from build123d import *

# Parameters (mm, degrees)
DOWELSUPPORT_DEPTH          = 1.905
DOWELSUPPORT_DEPTH_BACK     = 1.27
SKETCH3_R                   = 3.81
SKETCH5_W                   = 6.35
SKETCH5_H                   = 28.575
SLIDERDOWELSUPPORT_DEPTH    = 1.27
SLIDERDOWELCUTOUT_DEPTH     = 13.335
CUT_EXTRUDE2_DEPTH          = 29.782824115
CUT_EXTRUDE2_DEPTH_BACK     = 29.782824115
SKETCH20_W                  = 1.27
SKETCH20_H                  = 12.7
LPATTERN1_COUNT             = 2
LPATTERN1_PITCH             = 19.05
LATERALSUPPORT_DEPTH        = 1.27
SKETCH8_W                   = 6.35
SKETCH8_H                   = 3
TABSUPPORT_DEPTH            = 1.27
STRINGDOWELSUPPORT_START    = -1.27
STRINGDOWELSUPPORT_DEPTH    = 5.715
INTERSUPPORT_DEPTH          = 1.27
SKETCH10_W                  = 6.35
SKETCH10_H                  = 3
TABBASE_DEPTH               = 1.27
SKETCH12_W                  = 6.35
SKETCH12_H                  = 3
TABDRAFT_DEPTH              = 1.73
TABDRAFT_DRAFT              = 5
TABDRAFT_PROFILE_2_DEPTH    = 1.73
TABDRAFT_PROFILE_2_DRAFT    = 5
STRINGDOWELHOLES_DEPTH      = 39.922670163
STRINGDOWELHOLES_DEPTH_BACK = 1.524
SKETCH14_R                  = 1.600000102
PULLEYDOWELHOLE_DEPTH       = 2.921
FILLET1_R                   = 6.35


with BuildPart() as part:
    # Sketch3 → DowelSupport (new, two sides: drawn at the far end of the back side and taken through both)
    with BuildSketch(Plane(origin=(0, 0, 0), x_dir=(0, 0, -1), z_dir=(1, 0, 0)).offset(-DOWELSUPPORT_DEPTH_BACK)):
        with Locations((0, 24.60625)):
            Circle(SKETCH3_R)
    extrude(amount=DOWELSUPPORT_DEPTH + DOWELSUPPORT_DEPTH_BACK)

    # Sketch8 → TabSupport (add, symmetric)
    with BuildSketch(Plane(origin=(0, 0, 0), x_dir=(0, 0, -1), z_dir=(1, 0, 0))):
        with Locations((0, 21.59)):
            Rectangle(SKETCH8_W, SKETCH8_H)
        with Locations((-12.7, 21.59)):
            Rectangle(SKETCH8_W, SKETCH8_H)
    extrude(amount=TABSUPPORT_DEPTH, both=True)


with BuildPart() as body_2:
    # Sketch5 → SliderDowelSupport (new, symmetric)
    with BuildSketch(Plane(origin=(0, 0, 0), x_dir=(0, 0, -1), z_dir=(1, 0, 0))):
        Rectangle(SKETCH5_W, SKETCH5_H)
    extrude(amount=SLIDERDOWELSUPPORT_DEPTH, both=True)

    # Sketch19 → SliderDowelCutout (cut, symmetric)
    with BuildSketch(Plane(origin=(0, 0, 0), x_dir=(1, 0, 0), z_dir=(0, 1, 0))):
        with BuildLine():
            Line((1.27, 1.350000094), (1.243577144, 1.350000094))
            ThreePointArc((1.243577144, 1.350000094), (-1.068, 0), (1.243577144, -1.350000094))
            Line((1.243577144, -1.350000094), (1.27, -1.350000094))
            Line((1.27, -1.350000094), (1.27, 1.350000094))
        make_face()
    extrude(amount=SLIDERDOWELCUTOUT_DEPTH, both=True, mode=Mode.SUBTRACT)

    # Sketch20 → Cut-Extrude2 (cut, two sides: drawn at the far end of the back side and taken through both)
    with BuildSketch(Plane(origin=(1.27, 0, 0), x_dir=(0, 0, -1), z_dir=(1, 0, 0)).offset(-CUT_EXTRUDE2_DEPTH_BACK)):
        Rectangle(SKETCH20_W, SKETCH20_H)
    extrude(amount=CUT_EXTRUDE2_DEPTH + CUT_EXTRUDE2_DEPTH_BACK, mode=Mode.SUBTRACT)


with BuildPart() as lpattern1_1:
    # LPattern1: pattern copy
    add(body_2.part.moved(Location(Vector(0, 0, 1) * (1 * LPATTERN1_PITCH))))


with BuildPart() as body_4:
    # Sketch6 → LateralSupport (new, symmetric)
    with BuildSketch(Plane(origin=(0, 0, 0), x_dir=(0, 0, -1), z_dir=(1, 0, 0))):
        Polygon((7.392863577, 27.041434671), (5.805363577, 29.791065329), (8.169612929, 31.156065329), (9.523465192, 31.351124423), (10.602965192, 29.481375577), (9.757112929, 28.406434671), align=None)
    extrude(amount=LATERALSUPPORT_DEPTH, both=True)


with BuildPart() as tabsupport_piece_1:
    # of the separate pieces the step leaves, piece 1, a body of its own (tabsupport_pieces)
    add(part.part.solids().sort_by_distance((0, 24.60625, -3.81))[0])


with BuildPart() as tabsupport_piece_2:
    # of the separate pieces the step leaves, piece 2, a body of its own (tabsupport_pieces)
    add(part.part.solids().sort_by_distance((-1.27, 20.09, 9.525))[0])

    # Sketch15 → StringDowelSupport (add)
    with BuildSketch(Plane(origin=(0, 0, 0), x_dir=(0, 0, -1), z_dir=(1, 0, 0)).offset(STRINGDOWELSUPPORT_START)):
        with BuildLine():
            Line((-14.4145, 23.876), (-10.9855, 23.876))
            ThreePointArc((-10.9855, 23.876), (-8.6995, 21.59), (-10.9855, 19.304))
            Line((-10.9855, 19.304), (-14.4145, 19.304))
            ThreePointArc((-14.4145, 19.304), (-16.7005, 21.59), (-14.4145, 23.876))
        make_face()
    extrude(amount=STRINGDOWELSUPPORT_DEPTH)


with BuildPart() as body_2_1:
    add(body_2.part)

    add(lpattern1_1.part)  # InterSupport merges LPattern1_1

    add(body_4.part)  # InterSupport merges body 4

    add(tabsupport_piece_1.part)  # InterSupport merges TabSupport piece 1

    add(tabsupport_piece_2.part)  # InterSupport merges TabSupport piece 2
    # Sketch7 → InterSupport (add, symmetric)
    with BuildSketch(Plane(origin=(0, 0, 0), x_dir=(0, 0, -1), z_dir=(1, 0, 0))):
        Polygon((8.027863577, 25.941582409), (5.170363577, 30.890917591), (-1.187110053, 27.22042848), (-0.923046602, 27.310559749), (0, 24.60625), (1.42875, 22.131582409), align=None)
        Polygon((-1.42875, 27.080917591), (-1.187110053, 27.22042848), (-10.9855, 23.876), (-14.4145, 23.876), (-15.582507886, 22.531146949), (-22.225, 14.2875), (-15.875, 14.2875), (-15.875, 0), (-3.175, 0), (-3.175, 14.2875), (3.175, 14.2875), (3.175, 20.09), (0.923046602, 21.901940251), (0, 24.60625), align=None)
    extrude(amount=INTERSUPPORT_DEPTH, both=True)

    # Sketch10 → TabBase (add)
    with BuildSketch(Plane.ZY.offset(1.27)):
        with Locations((0, 21.59)):
            Rectangle(SKETCH10_W, SKETCH10_H)
        with Locations((12.7, 21.59)):
            Rectangle(SKETCH10_W, SKETCH10_H)
    extrude(amount=TABBASE_DEPTH)


with BuildPart() as tabdraft_tool:
    # Sketch12 → TabDraft (with draft: the straight prism first)
    with BuildSketch(Plane.ZY.offset(2.54)):
        with Locations((0, 21.59)):
            Rectangle(SKETCH12_W, SKETCH12_H)
    extrude(amount=TABDRAFT_DEPTH)
    # TabDraft: the draft: its side faces are tilted about the plane it starts from
    tabdraft_sides = [tabdraft_tool.faces().sort_by_distance(p)[0] for p in [
        (-3.405, 21.59, 3.175),
        (-3.405, 23.09, 0),
        (-3.405, 21.59, -3.175),
        (-3.405, 20.09, 0),
    ]]
    draft(tabdraft_sides, Plane.ZY.offset(2.54), TABDRAFT_DRAFT)


with BuildPart() as body_2_2:
    add(body_2_1.part)

    # TabDraft: add tabdraft_tool
    add(tabdraft_tool.part)


with BuildPart() as tabdraft_profile_2_tool:
    # Sketch12 → TabDraft profile 2 (with draft: the straight prism first)
    with BuildSketch(Plane.ZY.offset(2.54)):
        with Locations((12.7, 21.59)):
            Rectangle(SKETCH12_W, SKETCH12_H)
    extrude(amount=TABDRAFT_PROFILE_2_DEPTH)
    # TabDraft profile 2: the draft: its side faces are tilted about the plane it starts from
    tabdraft_profile_2_sides = [tabdraft_profile_2_tool.faces().sort_by_distance(p)[0] for p in [
        (-3.405, 21.59, 9.525),
        (-3.405, 20.09, 12.7),
        (-3.405, 21.59, 15.875),
        (-3.405, 23.09, 12.7),
    ]]
    draft(tabdraft_profile_2_sides, Plane.ZY.offset(2.54), TABDRAFT_PROFILE_2_DRAFT)


with BuildPart() as body_2_3:
    add(body_2_2.part)

    # TabDraft profile 2: add tabdraft_profile_2_tool
    add(tabdraft_profile_2_tool.part)

    # Sketch16 → StringDowelHoles (cut, two sides: drawn at the far end of the back side and taken through both)
    with BuildSketch(Plane(origin=(1.905, 0, 0), x_dir=(0, 0, -1), z_dir=(1, 0, 0)).offset(-STRINGDOWELHOLES_DEPTH_BACK)):
        with BuildLine():
            Line((-13.00760401, 20.828), (-12.39239599, 20.828))
            ThreePointArc((-12.39239599, 20.828), (-9.385499898, 21.59), (-12.39239599, 22.352))
            Line((-12.39239599, 22.352), (-13.00760401, 22.352))
            ThreePointArc((-13.00760401, 22.352), (-16.014500102, 21.59), (-13.00760401, 20.828))
        make_face()
    extrude(amount=STRINGDOWELHOLES_DEPTH + STRINGDOWELHOLES_DEPTH_BACK, mode=Mode.SUBTRACT)

    # Sketch14 → PulleyDowelHole (cut)
    with BuildSketch(Plane(origin=(1.905, 0, 0), x_dir=(0, 0, -1), z_dir=(1, 0, 0))):
        with Locations((0, 24.60625)):
            Circle(SKETCH14_R)
    extrude(amount=-PULLEYDOWELHOLE_DEPTH, mode=Mode.SUBTRACT)

    # Mirror1: body 2 across plane


with BuildPart() as body_2_4:
    add(body_2_3.part)
    add(body_2_3.part.mirror(Plane.ZX))

    # Fillet1
    fillet1_edges = [body_2_4.edges().sort_by_distance(p)[0] for p in [
        (0, -14.2875, 22.225),
        (0, 14.2875, 22.225),
    ]]
    fillet(fillet1_edges, radius=FILLET1_R)


solid = body_2_4.part
Can you work these out from the model? Positions are in its coordinate system, mm. A direction names the side the tool comes from. Coordinates: 2 decimals unless noted, no trailing zeros. Loops run counter-clockwise (first coordinate to the right, second up) from the corner with the lowest first, then second, coordinate; pieces in that order, holes last. Notation, with made-up numbers: (89.5, -17.75) - (120.5, -17.75) arc R14 cw to (120.5, 5.25) - close; hole circle Ø11 at (15, -14.75). An arc over 180 degrees is marked (long way). Put each result on its own line as item: value. Start each with the question number.
Item 1: Suppose I cut it at C-C (y = -7). Please give me the cut outline in (x, z) (3 decimals), and give its area (3 significant figures).
Item 2: Suppose I cut it at D-D (z = 15). Please give me the cut outline in (x, y) (3 decimals), and give its area (3 significant figures).
Item 3: For pin 1 (1 mm diameter, centred on x = -2, y = 22, fed in from +Z) (3 decimals); pin 2 (1.4 mm diameter, centred on x = -2, z = 1.5, fed in from -Y); pin 3 (6 mm diameter, centred on y = 25, z = 1, fed in from +X) (3 decimals), each with a flat end and sliding along its axis, tell me the tip position at first contact or that it passes through.
Item 4: Suppose I cut it at B-B (z = 19.05). Please give me the cut outline in (x, y) (3 decimals).
Item 5: Which directions (+Z, -Z, +X, -X, +Y, -Y) give clear straight access to the entire face, cutting with the end or side of a thin tool? Please do faces 1 (the face through (2, -23.876, 13)), 2 (the face through (0.018, -30.333, -5.492)), 3 (the face through (-2, 20.09, 0)), 4 (the face through (1.905, -25, -2)).
Item 6: If I drill on line 1 along Y through (x, z) = (-2.5, 0.5); line 2 along Z through (x, y) = (2, -22.5); line 3 along Z through (x, y) = (1.4, -21.59), over which ranges is the centre line in solid material (lowest first)?
Item 7: If we mould it in two halves opening along Y, with no side actions, what happens to faces 5 (the face through (0.018, 25.205, 7.093)), 6 (the face through (2.8, 21.6, 8.7)), 7 (the face through (0, -13.335, 0)), 8 (the face through (4.445, -20.6, 12.6))? For each: +Y half, -Y half, draft (parallel to the pull), parting line (faces both ways), or undercut.
Item 8: Suppose I cut it at A-A (x = 2.5). Please give me the cut outline in (y, z).
Here are the results:
1. outline: (-1.27, -3.175) - (1.27, -3.175) - (1.27, -1.35) - (1.244, -1.35) arc R1.55 cw (long way) to (1.244, 1.35) - (1.27, 1.35) - (1.27, 17.7) - (1.244, 17.7) arc R1.55 cw (long way) to (1.244, 20.4) - (1.27, 20.4) - (1.27, 22.225) - (-1.27, 22.225) - close
1. area: 52.3 mm²
2. outline: (-4.27, -22.939) - (-2.54, -23.09) - (-1.27, -23.09) - (-1.27, -23.8) - (4.445, -23.8) - (4.445, -23.079) - (0.381, -23.079) - (0.381, -20.101) - (4.445, -20.101) - (4.445, -19.38) - (1.27, -19.38) - (1.27, 19.38) - (4.445, 19.38) - (4.445, 20.101) - (0.381, 20.101) - (0.381, 23.079) - (4.445, 23.079) - (4.445, 23.8) - (-1.27, 23.8) - (-1.27, 23.09) - (-2.54, 23.09) - (-4.27, 22.939) - (-4.27, 20.241) - (-2.54, 20.09) - (-1.27, 20.09) - (-1.27, -20.09) - (-2.54, -20.09) - (-4.27, -20.241) - close
2. area: 142 mm²
3. pin 1: z = 15.875
3. pin 2: y = -23.09
3. pin 3: x = 1.905
4. outline: (-1.27, -18.228) - (1.27, -18.228) - (1.27, -13.335) - (-1.068, -13.335) - (-1.068, -6.35) - (-1.27, -6.35) - close; (-1.27, 6.35) - (-1.068, 6.35) - (-1.068, 13.335) - (1.27, 13.335) - (1.27, 18.228) - (-1.27, 18.228) - close
5. face 1: +Z, +X, -X, -Y
5. face 2: +X, -X, -Y
5. face 3: +Z, -Z, -X
5. face 4: -Z, +X, +Y, -Y
6. line 1: -23.09 to -20.09, 20.09 to 23.09
6. line 2: 8.89 to 9.67, 12.3 to 13.1, 15.73 to 16.51
6. line 3: -2.33 to 2.33, 8.7 to 9.39, 16.01 to 16.7
7. face 5: +Y half
7. face 6: undercut
7. face 7: undercut
7. face 8: draft
8. outline: (-23.88, 10.99) arc R2.29 ccw to (-19.3, 10.99) - (-19.3, 14.41) arc R2.29 ccw to (-23.88, 14.41) - close; (19.3, 10.99) arc R2.29 ccw to (23.88, 10.99) - (23.88, 14.41) arc R2.29 ccw to (19.3, 14.41) - close; hole (-22.35, 12.39) arc R1.6 ccw (long way) to (-20.83, 12.39) - (-20.83, 13.01) arc R1.6 ccw (long way) to (-22.35, 13.01) - close; hole (20.83, 12.39) arc R1.6 ccw (long way) to (22.35, 12.39) - (22.35, 13.01) arc R1.6 ccw (long way) to (20.83, 13.01) - close
